The listing builds one solid part. Answer for the finished solid, in the listing's coordinates (mm). Face numbers are marked on the shaded views. A direction names the side the tool comes from. Round coordinates to 2 decimals unless told otherwise and drop trailing zeros. Loops run counter-clockwise (first coordinate to the right, second up) from the corner with the lowest first, then second, coordinate; pieces in that order, holes last. Notation, with made-up numbers: (24, 65.5) -> (57, 65.5) arc R20 cw to (57, 84.5) -> close; hole circle Ø8 at (9, 24.5). An arc over 180 degrees is marked (long way). Write each question's results on one line, items separated by ' | '. Start each with the question number.
(1) The part is cut by section A-A (x = -2.5). Determine the outline of the cut face in (y, z), plus the area to 3 significant figures.
(2) Determine the mould class of the marked faces 1, 2 and 3 for opening direction X: released by +X, released by -X, zero draft, split by the parting line, or undercut.
(3) Flat-ended cylindrical pins translate along their axes: pin 1 (1.5 mm diameter, centred on y = -1.5, z = 3, fed in from -X); pin 2 (1 mm diameter, centred on y = 0.5, z = 1, fed in from +X); pin 3 (4 mm diameter, centred on y = 0.5, z = 13.5, fed in from +X). Find the tip coordinate at first contact, or state that the pin passes through.
(4) The part is cut by section C-C (y = -2). Determine the outline of the cut face in (x, z), plus the area to 3 significant figures.
(5) The part is cut by section B-B (z = 1.25). Determine the outline of the cut face in (x, y).
(6) Straight lines are drawn through the part: probe 1 along Y at (x, z) = (-7.5, 10.5); probe 2 along Z at (x, y) = (18, 1.5); probe 3 along Z at (x, y) = (8.5, -4.5). For each, find the intervals that lie inside material, in ascending order.
(7) For the marked faces 4, 5, 6 and 7, determine the directions among +Z, -Z, +X, -X, +Y, -Y from which every point of the face is accessible in a straight line to the end or side of a thin tool.
(8) The part is cut by section D-D (z = 3.5). Determine the outline of the cut face in (x, y), plus the area to 3 significant figures.
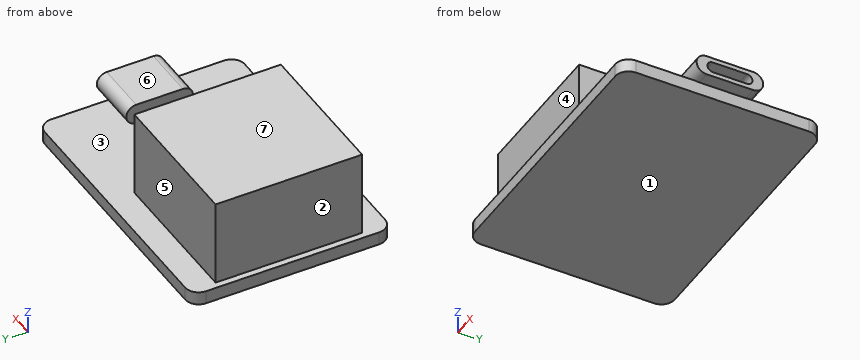
Autodesk Inventor part; units mm, degrees
ref_plane "YZ Plane" through (0, 0, 0) normal (1, 0, 0) x (0, 1, 0)
ref_plane "XZ Plane" through (0, 0, 0) normal (0, 1, 0) x (-1, 0, 0)
ref_plane "XY Plane" through (0, 0, 0) normal (0, 0, 1) x (1, 0, 0)
sketch "草图1" plane through (0, 0, 0) normal (0, 0, 1) x (1, 0, 0)
  line L0 (21, -15) -> (-21, -15)
  line L1 (-21, -15) -> (-21, 15)
  line L2 (-21, 15) -> (21, 15)
  line L3 (21, 15) -> (21, -15)
  line L4 (21, -15) -> (-21, 15) construction
  line L5 (-21, -15) -> (21, 15) construction
  point P0 (0, 0)
  dimension "d0" = 42
  dimension "d1" = 30
extrude "拉伸1" add sketch "草图1" along normal blind 2
sketch "草图2" plane through (0, 0, 2) normal (0, 0, 1) x (1, 0, 0)
  line L0 (2, -11) -> (-20, -11)
  line L1 (-20, -11) -> (-20, 11)
  line L2 (-20, 11) -> (2, 11)
  line L3 (2, 11) -> (2, -11)
  line L4 (2, -11) -> (-20, 11) construction
  line L5 (-20, -11) -> (2, 11) construction
  line L6 (-21, 15) -> (-21, -15)
  point P0 (0, 0)
  point P1 (-9, 0)
  dimension "d4" = 22
  dimension "d5" = 22
  dimension "d6" = 1
extrude "拉伸2" add sketch "草图2" along normal blind 13
sketch "草图3" plane through (0, 0, 2) normal (0, 0, 1) x (1, 0, 0)
  point P0 (0, 0)
sketch "草图4" plane through (21, -15, 0) normal (1, 0, 0) x (0, 0, -1)
  line L0 (0, 15) -> (-5.9619, 15)
  line L1 (-3.4523, 11.5) -> (-3.4523, 18.5) construction
  line L2 (-1.9523, 11.5) -> (-1.9523, 18.5)
  line L3 (-4.9523, 18.5) -> (-4.9523, 11.5)
  arc A0 (-4.9523, 11.5) -> (-1.9523, 11.5) centre (-3.4523, 11.5) ccw
  arc A1 (-1.9523, 18.5) -> (-4.9523, 18.5) centre (-3.4523, 18.5) ccw
  line L4 (-3.4523, 12.4289) -> (-3.4523, 17.5711) construction
  line L5 (-2.6459, 12.4289) -> (-2.6459, 17.5711)
  line L6 (-4.2587, 17.5711) -> (-4.2587, 12.4289)
  arc A2 (-4.2587, 12.4289) -> (-2.6459, 12.4289) centre (-3.4523, 12.4289) ccw
  arc A3 (-2.6459, 17.5711) -> (-4.2587, 17.5711) centre (-3.4523, 17.5711) ccw
  point P0 (-3.4523, 15)
  point P1 (-3.4523, 10)
  point P2 (-3.4523, 20)
  dimension "d9" = 3
  dimension "d10" = 10
extrude "拉伸3" add sketch "草图4" against normal blind 6 contours L2 A0 L3 L0 L6 A2 L5 | L0 L5 A3 L6 L3 A1 L2
extrude "拉伸4" add sketch "草图4" along normal blind 2 contours L2 A0 L3 L0 L6 A2 L5 | L0 L5 A3 L6 L3 A1 L2
sketch "草图5" plane through (15, -15, 0) normal (-1, 0, 0) x (0, 0, 1)
  line L0 (2.6459, 12.4289) -> (2.6459, 17.5711)
  arc A0 (4.2587, 17.5711) -> (2.6459, 17.5711) centre (3.4523, 17.5711) ccw
  line L1 (4.2587, 17.5711) -> (4.2587, 12.4289)
  arc A1 (2.6459, 12.4289) -> (4.2587, 12.4289) centre (3.4523, 12.4289) ccw
  line L2 (2, 11.1247) -> (2, 18.8753)
  arc A2 (2, 11.1247) -> (4.9523, 11.5) centre (3.4523, 11.5) ccw
  line L3 (4.9523, 11.5) -> (4.9523, 18.5)
  arc A3 (4.9523, 18.5) -> (2, 18.8753) centre (3.4523, 18.5) ccw
  point P0 (0, 15)
extrude "拉伸5" add sketch "草图5" against normal blind 4.25 contours L0 A0 L1 A1 | L2 A3 L3 A2
fillet "圆角1" radius 2 4 edges at (21, -15, 1) (-21, -15, 1) (21, 15, 1) (-21, 15, 1)
properties part number "陀螺仪"
Checked values:
1) outline: (-15, 0) -> (15, 0) -> (15, 2) -> (11, 2) -> (11, 15) -> (-11, 15) -> (-11, 2) -> (-15, 2) -> close | area: 346 mm2
2) face 1: zero draft | face 2: released by -X | face 3: undercut
3) pin 1: stops at x = -20 | pin 2: stops at x = 21 | pin 3: stops at x = 2
4) outline: (-21, 0) -> (21, 0) -> (21, 1.95) -> (23, 1.95) -> (23, 2.65) -> (19.25, 2.65) -> (19.25, 4.26) -> (23, 4.26) -> (23, 4.95) -> (15, 4.95) -> (15, 2) -> (2, 2) -> (2, 15) -> (-20, 15) -> (-20, 2) -> (-21, 2) -> close | area: 388 mm2
5) outline: (-21, -13) arc R2 ccw to (-19, -15) -> (19, -15) arc R2 ccw to (21, -13) -> (21, 13) arc R2 ccw to (19, 15) -> (-19, 15) arc R2 ccw to (-21, 13) -> close
6) probe 1: y = -11 to 11 | probe 2: z = 0 to 4.95 | probe 3: z = 0 to 2
7) face 4: +Z, +X, -X, -Y | face 5: +Z, +X, -X, +Y | face 6: +Z, +X, +Y, -Y | face 7: +Z, +X, -X, +Y, -Y
8) outline: (-20, -11) -> (2, -11) -> (2, 11) -> (-20, 11) -> close; (15, -5) -> (23, -5) -> (23, -3.38) -> (19.25, -3.38) -> (19.25, 3.38) -> (23, 3.38) -> (23, 5) -> (15, 5) -> close | area: 539 mm2
